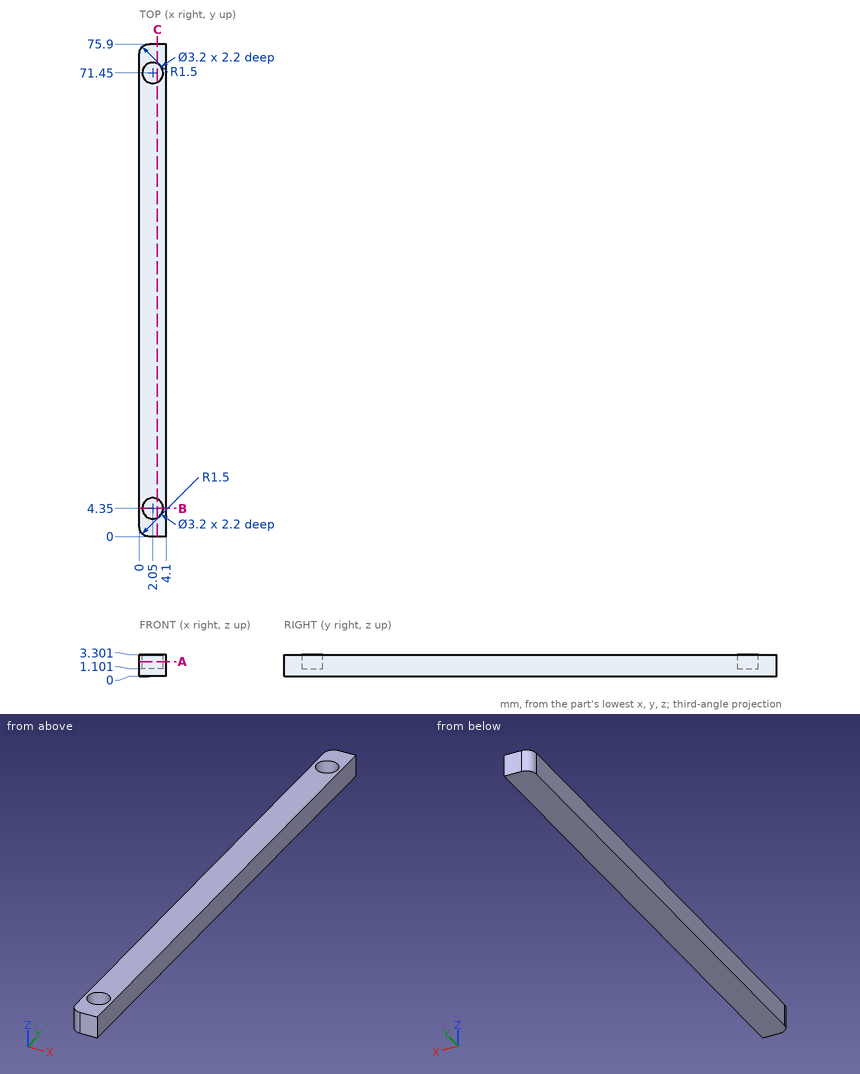
The drawing under review shows one solid part. Ordinate dimensions are in mm from its lowest x, y, z. Round coordinates to 2 decimals unless told otherwise and drop trailing zeros. Write each loop counter-clockwise with the first axis right and the second up, starting at its lowest first coordinate (ties: lowest second). Pieces come first, ordered by that corner, then holes. Notation, with made-up numbers: (-31.75, 6) -> (-14.75, 6) arc R31 ccw to (-14.75, 31) -> close; hole circle Ø7 at (5, 61.25). An arc over 180 degrees is marked (long way). One line per question, with ' | ' between items. Start each with the question number.
(1) Add section A-A, the plane z = 2.2. Write out the cut boundary in (x, y), plus the area to 3 significant figures.
(2) Insertion check: P1, Ø1.6, axis at x = 2, y = 4, coming from the +Z side. The pin has a flat end and moves straight along its axis. Give the tip position at first contact, or say it passes through.
(3) Add section B-B, the plane y = 4.35. Write out the cut boundary in (x, z).
(4) Add section C-C, the plane x = 2.75. Write out the cut boundary in (y, z).
(5) For line 1 along X through (y, z) = (71.45, 1.95); line 2 along Y through (x, z) = (1.25, 2.1) (1 decimal); line 3 along Y through (x, z) = (3.15, 2.4), list the stretches that pass through material, from the lowest coordinate up. Write a range as from..to.
Answer list:
1) outline: (0, 1.5) arc R1.5 ccw to (1.5, 0) -> (4.1, 0) -> (4.1, 75.9) -> (1.5, 75.9) arc R1.5 ccw to (0, 74.4) -> close; hole circle Ø3.2 at (2.05, 4.35); hole circle Ø3.2 at (2.05, 71.45) | area: 294 mm²
2) P1: z = 1.1
3) outline: (0, 0) -> (4.1, 0) -> (4.1, 3.3) -> (3.65, 3.3) -> (3.65, 1.1) -> (0.45, 1.1) -> (0.45, 3.3) -> (0, 3.3) -> close
4) outline: (0, 0) -> (75.9, 0) -> (75.9, 3.3) -> (72.89, 3.3) -> (72.89, 1.1) -> (70.01, 1.1) -> (70.01, 3.3) -> (5.79, 3.3) -> (5.79, 1.1) -> (2.91, 1.1) -> (2.91, 3.3) -> (0, 3.3) -> close
5) line 1: 0..0.45, 3.65..4.1 | line 2: 0..3, 5.7..70.1, 72.8..75.9 | line 3: 0..3.19, 5.51..70.29, 72.61..75.9
